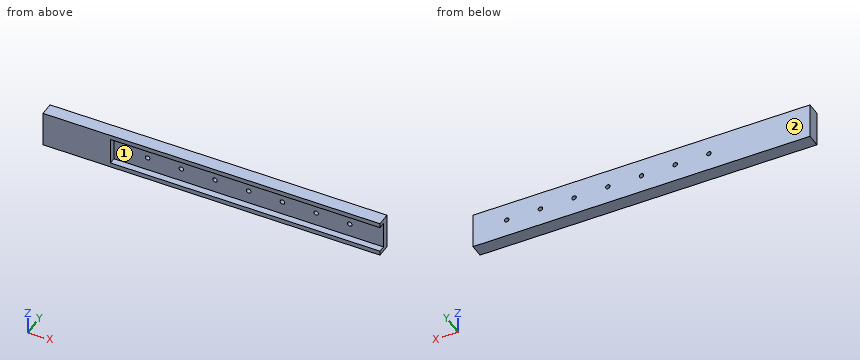
from build123d import *

# Parameters (mm, degrees)
IZIM2_W                     = 750
IZIM2_H                     = 80
IZIM2_R                     = 5
Y_KSEKLIK_EKSTR_ZYON1_DEPTH = 30
IZIM3_W                     = 60
IZIM3_H                     = 15
KES_EKSTR_ZYON1_DEPTH       = 600


with BuildPart() as part:
    # Çizim2 → Yükseklik-Ekstrüzyon1 (new body)
    with BuildSketch(Plane(origin=(0, 0, 0), x_dir=(1, 0, 0), z_dir=(0, 1, 0))):
        Rectangle(IZIM2_W, IZIM2_H)
        with Locations((300, 0)):
            Circle(IZIM2_R, mode=Mode.SUBTRACT)
        with Locations((225, 0)):
            Circle(IZIM2_R, mode=Mode.SUBTRACT)
        with Locations((150, 0)):
            Circle(IZIM2_R, mode=Mode.SUBTRACT)
        with Locations((75, 0)):
            Circle(IZIM2_R, mode=Mode.SUBTRACT)
        Circle(IZIM2_R, mode=Mode.SUBTRACT)
        with Locations((-75, 0)):
            Circle(IZIM2_R, mode=Mode.SUBTRACT)
        with Locations((-150, 0)):
            Circle(IZIM2_R, mode=Mode.SUBTRACT)
    extrude(amount=-Y_KSEKLIK_EKSTR_ZYON1_DEPTH)

    # Çizim3 → Kes-Ekstrüzyon1 (cut)
    with BuildSketch(Plane(origin=(375, 0, 0), x_dir=(0, 0, -1), z_dir=(1, 0, 0))):
        with Locations((0, -22.5)):
            Rectangle(IZIM3_W, IZIM3_H)
    extrude(amount=-KES_EKSTR_ZYON1_DEPTH, mode=Mode.SUBTRACT)


solid = part.part
Design review of the part built by this model. Coordinates are the model's own, in mm. Face numbers are marked on the shaded views. A direction names the side the tool comes from. Round coordinates to 2 decimals unless told otherwise and drop trailing zeros. Write each loop counter-clockwise with the first axis right and the second up, starting at its lowest first coordinate (ties: lowest second). Pieces come first, ordered by that corner, then holes.
Item 1: For the marked faces 1 and 2, list the 3-axis set-ups (+Z, -Z, +X, -X, +Y, -Y) from which the entire face can be reached by the end or side of a thin tool; tool diameter is ignored.
Item 2: Consider section A-A on z = -17. Give the boundary of the cut face in (x, y), and give its area (3 significant figures).
Item 3: Wall thickness on L1, parallel to Z at x = 225, y = -7.75; L2, parallel to Z at x = 89.5, y = -20; L3, parallel to X at y = -28, z = 11: over which ranges is each line inside the solid? List them lowest first.
Item 4: For pin 1 Ø12 at (x, z) = (42, 7.5) entering from +Y; pin 2 Ø1.5 at (x, z) = (68.5, 22) entering from -Y; pin 3 Ø1 at (y, z) = (-26.5, -9) entering from +X; pin 4 Ø6 at (x, z) = (75, 0) entering from +Y, all flat-tipped, find the tip position at first contact; note any pin that passes through.
Check values:
1. face 1: +X, -Y
1. face 2: +Z, -Z, +X, -X, +Y
2. outline: (-375, -30) - (-225, -30) - (-225, -15) - (375, -15) - (375, 0) - (-375, 0) - close
2. area: 13,500 mm2
3. L1: z = -40 to -5, 5 to 40
3. L2: z = -40 to -30, 30 to 40
3. L3: x = -375 to -225
4. pin 1: stops at y = 0
4. pin 2: stops at y = -15
4. pin 3: stops at x = -225
4. pin 4: passes through
